Geometry: final body of the model. Coordinates: model frame, mm. Face numbers are marked on the shaded views. A direction names the side the tool comes from. Give positions to 0.01 mm unless a question says otherwise; leave off trailing zeros. Write each loop counter-clockwise with the first axis right and the second up, starting at its lowest first coordinate (ties: lowest second). Pieces come first, ordered by that corner, then holes. Notation, with made-up numbers: (-2.75, 51) - (55.25, 51) arc R9 ccw to (55.25, 55) - close; hole circle Ø8 at (45, 24). An arc over 180 degrees is marked (long way). One line per question, with ' | ' between items. Start each with the question number.
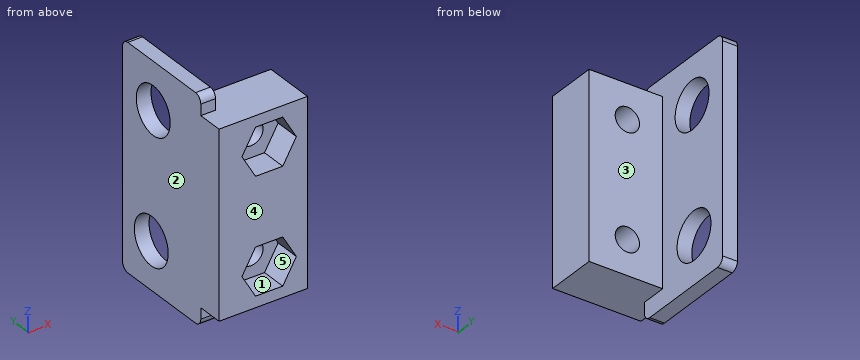
```python
from build123d import *

# Parameters (mm, degrees)
SKETCH1_W           = 12
SKETCH1_H           = 25
SKETCH1_R           = 1.65
BOSS_EXTRUDE1_DEPTH = 3.5
CUT_EXTRUDE1_DEPTH  = 3.5
SKETCH3_R           = 3.25
BOSS_EXTRUDE2_DEPTH = 2


with BuildPart() as part:
    # Sketch1 → Boss-Extrude1 (new, symmetric)
    with BuildSketch(Plane(origin=(0, 0, 0), x_dir=(1, 0, 0), z_dir=(0, 1, 0))):
        Rectangle(SKETCH1_W, SKETCH1_H)
        with Locations(Location((0.804958277, -7.8, 0), (0, 0, 270))):
            Circle(SKETCH1_R, mode=Mode.SUBTRACT)
        with Locations(Location((0.804958277, 7.8, 0), (0, 0, 90))):
            Circle(SKETCH1_R, mode=Mode.SUBTRACT)
    extrude(amount=BOSS_EXTRUDE1_DEPTH, both=True)

    # Sketch2 → Cut-Extrude1 (cut)
    with BuildSketch(Plane.XZ.offset(3.5)):
        Polygon((2.652479139, 4.6), (4.5, 7.8), (2.652479139, 11), (-1.042562584, 11), (-2.890083446, 7.8), (-1.042562584, 4.6), align=None)
        Polygon((2.652479139, -11), (4.5, -7.8), (2.652479139, -4.6), (-1.042562584, -4.6), (-2.890083446, -7.8), (-1.042562584, -11), align=None)
    extrude(amount=-CUT_EXTRUDE1_DEPTH, mode=Mode.SUBTRACT)

    # Sketch3 → Boss-Extrude2 (add)
    with BuildSketch(Plane.ZY.offset(6)):
        with BuildLine():
            Line((0, 0), (14, 0))
            ThreePointArc((14, 0), (14.707106781, 0.292893219), (15, 1))
            Line((15, 1), (15, 14))
            ThreePointArc((15, 14), (14.707106781, 14.707106781), (14, 15))
            Line((14, 15), (-14, 15))
            ThreePointArc((-14, 15), (-14.707106781, 14.707106781), (-15, 14))
            Line((-15, 14), (-15, 1))
            ThreePointArc((-15, 1), (-14.707106781, 0.292893219), (-14, 0))
            Line((-14, 0), (0, 0))
        make_face()
        with Locations((-8.581197846, 9.5)):
            Circle(SKETCH3_R, mode=Mode.SUBTRACT)
        with Locations((8.581197846, 9.124939365)):
            Circle(SKETCH3_R, mode=Mode.SUBTRACT)
    extrude(amount=-BOSS_EXTRUDE2_DEPTH)


solid = part.part
```
1) Section A-A, the plane y = -2. Output: boundary loops of the cut face in (x, z).
2) Section B-B, the plane x = 1.5. Output: boundary loops of the cut face in (y, z), plus the area to 3 significant figures.
3) First-contact query: pin 1 Ø3 at (x, y) = (1.5, -1) entering from -Z; pin 2 Ø1.8 at (x, y) = (0, -2) entering from +Z; pin 3 Ø3 at (x, z) = (-1, 0) entering from +Y; pin 4 Ø4 at (y, z) = (9.5, -8.58) entering from -X. Flat tips, straight axial feed; report the tip coordinate or a pass-through.
4) Pull-direction query (Z, two-part tool) for the marked faces 4 and 5; classes: +Z half, -Z half, draft (parallel to the pull), parting line (faces both ways), or undercut.
5) Section D-D, the plane z = -3. Output: boundary loops of the cut face in (x, y).
6) Section C-C, the plane y = 9.5. Output: boundary loops of the cut face in (x, z).
7) Line query: L1, parallel to Z at x = -1, y = -1.25; L2, parallel to X at y = 1.75, z = 7.8; L3, parallel to Z at x = 5, y = -0.25. Output: solid intervals per line, ascending.
8) Reachability of the marked faces 1, 2 and 3 from +Z, -Z, +X, -X, +Y, -Y: full face, straight path, thin tool, end or side. Return the list, or none.
Answer key:
1) outline: (-6, -12.5) - (6, -12.5) - (6, 12.5) - (-6, 12.5) - close; hole (-2.89, -7.8) - (-1.04, -11) - (2.65, -11) - (4.5, -7.8) - (2.65, -4.6) - (-1.04, -4.6) - close; hole (-2.89, 7.8) - (-1.04, 4.6) - (2.65, 4.6) - (4.5, 7.8) - (2.65, 11) - (-1.04, 11) - close
2) outline: (-3.5, -12.5) - (3.5, -12.5) - (3.5, -9.3) - (0, -9.3) - (0, -11) - (-3.5, -11) - close; (-3.5, -4.6) - (0, -4.6) - (0, -6.3) - (3.5, -6.3) - (3.5, 6.3) - (0, 6.3) - (0, 4.6) - (-3.5, 4.6) - close; (-3.5, 11) - (0, 11) - (0, 9.3) - (3.5, 9.3) - (3.5, 12.5) - (-3.5, 12.5) - close | area: 109 mm^2
3) pin 1: z = -12.5 | pin 2: z = 12.5 | pin 3: y = 3.5 | pin 4: through
4) face 4: draft | face 5: undercut
5) outline: (-6, -3.5) - (6, -3.5) - (6, 3.5) - (-4, 3.5) - (-4, 15) - (-6, 15) - close
6) outline: (-6, -15) - (-4, -15) - (-4, -11.83) - (-6, -11.83) - close; (-6, -5.33) - (-4, -5.33) - (-4, 5.35) - (-6, 5.35) - close; (-6, 11.81) - (-4, 11.81) - (-4, 15) - (-6, 15) - close
7) L1: -12.5 to -11, -4.6 to 4.6, 11 to 12.5 | L2: -6 to -0.85, 2.45 to 6 | L3: -12.5 to 12.5
8) face 1: -Y | face 2: +Z, -Z, -X, +Y, -Y | face 3: +Z, -Z, +X, +Y
